For this review, use the dimensioned drawing (mm, ordinates from the lowest corner) and the shaded views. A direction names the side the tool comes from. Coordinates: 2 decimals unless noted, no trailing zeros. Order: outer loops, then holes, each group sorted by start corner. A loop starts at its lowest first (then second) coordinate and runs counter-clockwise, first axis right, second up. Notation, with made-up numbers: M 70,16 L 113,16 A24 cw 113,40 Z; hole C 37.25,-27 d7. An arc over 180 degrees is marked long. One line per item, written item: value.
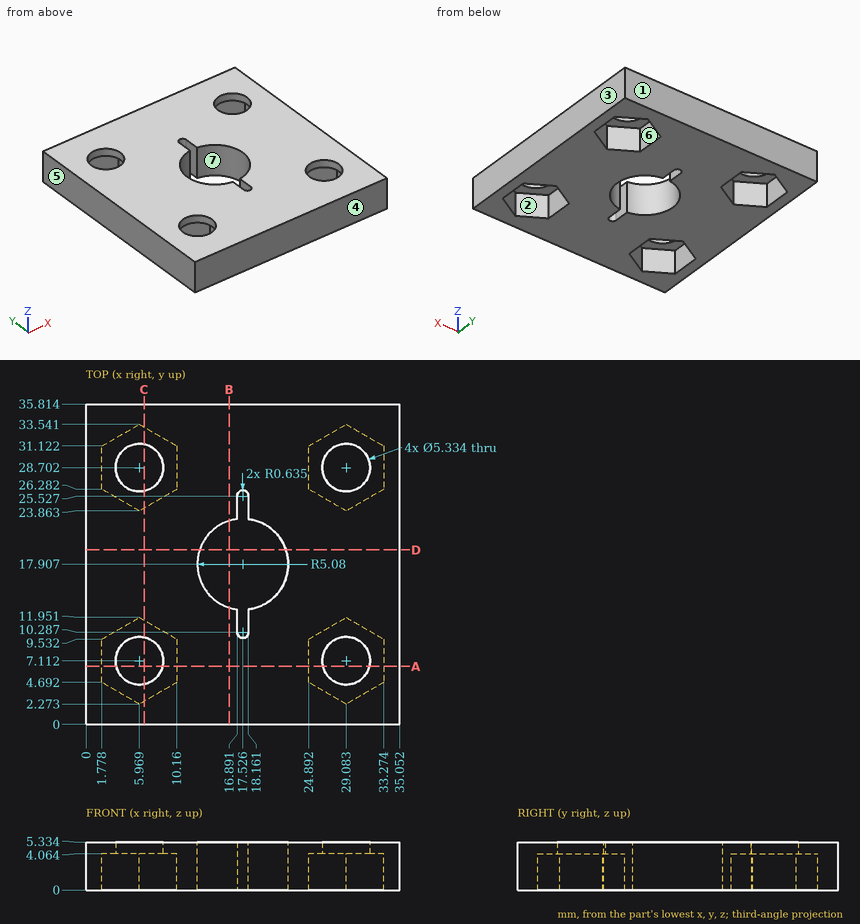
(1) We need section C-C, the plane x = 6.5. State the section outline as (y, z) points (1 decimal).
Geometry results:
outline: M 0,0 L 2.6,0 L 2.6,4.1 L 4.5,4.1 L 4.5,5.3 L 0,5.3 Z; M 9.7,4.1 L 11.6,4.1 L 11.6,0 L 24.2,0 L 24.2,4.1 L 26.1,4.1 L 26.1,5.3 L 9.7,5.3 Z; M 31.3,4.1 L 33.2,4.1 L 33.2,0 L 35.8,0 L 35.8,5.3 L 31.3,5.3 Z
(2) Tool access review of the marked faces 5, 6 and 7: name each direction out of +Z, -Z, +X, -X, +Y, -Y from which nothing blocks a thin tool from reaching the whole face with its end or side.
Geometry results:
face 5: +Z, -Z, -X, +Y, -Y
face 6: -Z
face 7: +Z, -Z
(3) We need section A-A, the plane y = 6.5. State the section outline as (x, z) points (1 decimal).
Geometry results:
outline: M 0,0 L 1.8,0 L 1.8,4.1 L 3.4,4.1 L 3.4,5.3 L 0,5.3 Z; M 8.6,4.1 L 10.2,4.1 L 10.2,0 L 24.9,0 L 24.9,4.1 L 26.5,4.1 L 26.5,5.3 L 8.6,5.3 Z; M 31.7,4.1 L 33.3,4.1 L 33.3,0 L 35.1,0 L 35.1,5.3 L 31.7,5.3 Z
(4) We need section D-D, the plane y = 19.5. State the section outline as (x, z) points.
Geometry results:
outline: M 0,0 L 12.7,0 L 12.7,5.33 L 0,5.33 Z; M 22.35,0 L 35.05,0 L 35.05,5.33 L 22.35,5.33 Z
(5) Mouldability with a two-part tool opening along Y and no side actions: class the marked faces 1, 2, 3 and 4 as +Y half, -Y half, draft (parallel to the pull), parting line (faces both ways), or undercut.
Geometry results:
face 1: +Y half
face 2: undercut
face 3: draft
face 4: -Y half
(6) We need section B-B, the plane x = 16. State the section outline as (y, z) points, plus the area to 3 significant figures.
Geometry results:
outline: M 0,0 L 13.06,0 L 13.06,5.33 L 0,5.33 Z; M 22.75,0 L 35.81,0 L 35.81,5.33 L 22.75,5.33 Z
area: 139 mm2
(7) For L1, parallel to X at y = 30, z = 0.35; L2, parallel to X at y = 28.5, z = 4.4; L3, parallel to Y at x = 29, z = 4.1, list the stretches that pass through material, from the lowest coordinate up.
Geometry results:
L1: x = 0 to 1.78, 10.16 to 24.89, 33.27 to 35.05
L2: x = 0 to 3.31, 8.63 to 26.42, 31.74 to 35.05
L3: y = 0 to 4.45, 9.78 to 26.04, 31.37 to 35.81
(8) Insertion check: pin 1 Ø3 at (x, z) = (19.5, 1.5) entering from -Y. The pin has a flat end and moves straight along its axis. Give the tip position at first contact, or say it passes through.
Geometry results:
pin 1: stops at y = 0
